The model under review builds one solid part; all positions refer to its coordinate system, in mm. Face numbers are marked on the shaded views. A direction names the side the tool comes from. Give positions to 0.01 mm unless a question says otherwise; leave off trailing zeros. Loops run counter-clockwise (first coordinate to the right, second up) from the corner with the lowest first, then second, coordinate; pieces in that order, holes last. Notation, with made-up numbers: (46.5, 54.25) - (88.5, 54.25) arc R22 cw to (88.5, 60.25) - close; hole circle Ø10 at (-26.5, 71.25). An arc over 180 degrees is marked (long way). Return JSON: item names as keys, results as strings. Group by question number.
from build123d import *

# Parameters (mm, degrees)
SKETCH1_W           = 23
SKETCH1_H           = 12
BOSS_EXTRUDE1_DEPTH = 32
SKETCH2_W           = 4.5
SKETCH2_H           = 2
BOSS_EXTRUDE2_DEPTH = 12
CUT_EXTRUDE1_DEPTH  = 37.912057651
SKETCH4_W           = 23
SKETCH4_H           = 12
SKETCH4_R           = 2.5
CUT_EXTRUDE2_DEPTH  = 3.5
CUT_EXTRUDE3_DEPTH  = 5.5
FILLET1_R           = 1


with BuildPart() as part:
    # Sketch1 → Boss-Extrude1 (new body)
    with BuildSketch(Plane.XY):
        with Locations((11.5, 6)):
            Rectangle(SKETCH1_W, SKETCH1_H)
    extrude(amount=BOSS_EXTRUDE1_DEPTH)

    # Sketch2 → Boss-Extrude2 (add)
    with BuildSketch(Plane.XZ):
        with Locations((-2.25, 20.5)):
            Rectangle(SKETCH2_W, SKETCH2_H)
        with Locations((25.25, 20.5)):
            Rectangle(SKETCH2_W, SKETCH2_H)
    extrude(amount=-BOSS_EXTRUDE2_DEPTH)

    # Sketch3 → Cut-Extrude1 (cut, through all)
    with BuildSketch(Plane.XY.offset(21.5)):
        with BuildLine():
            Line((-3.549038106, 6.75), (-4.5, 6.75))
            Line((-4.5, 6.75), (-4.5, 5.25))
            Line((-4.5, 5.25), (-3.549038106, 5.25))
            ThreePointArc((-3.549038106, 5.25), (-0.75, 6), (-3.549038106, 6.75))
        make_face()
        with BuildLine():
            Line((26.549038106, 6.75), (27.5, 6.75))
            Line((27.5, 6.75), (27.5, 5.25))
            Line((27.5, 5.25), (26.549038106, 5.25))
            ThreePointArc((26.549038106, 5.25), (23.75, 6), (26.549038106, 6.75))
        make_face()
    extrude(amount=-CUT_EXTRUDE1_DEPTH, mode=Mode.SUBTRACT)

    # Sketch4 → Cut-Extrude2 (cut)
    with BuildSketch(Plane.XY.offset(32)):
        with Locations((11.5, 6)):
            Rectangle(SKETCH4_W, SKETCH4_H)
        with Locations((6, 6)):
            Circle(SKETCH4_R, mode=Mode.SUBTRACT)
    extrude(amount=-CUT_EXTRUDE2_DEPTH, mode=Mode.SUBTRACT)

    # Sketch5 → Cut-Extrude3 (cut)
    with BuildSketch(Plane.XY.offset(28.5)):
        with BuildLine():
            ThreePointArc((11.479166667, 3.554855293), (9.2656647, 0.966568361), (6.000000021, 0))
            Line((6.000000021, 0), (23, 0))
            Line((23, 0), (23, 12))
            Line((23, 12), (6.000000023, 12))
            ThreePointArc((6.000000023, 12), (9.265664701, 11.033431639), (11.479166667, 8.445144707))
            ThreePointArc((11.479166667, 8.445144707), (14.5, 6), (11.479166667, 3.554855293))
        make_face()
        with BuildLine():
            Line((0, 12), (0, 6.000000008))
            ThreePointArc((0, 6.000000008), (1.757359324, 10.242640698), (6.000000023, 12))
            Line((6.000000023, 12), (0, 12))
        make_face()
        with BuildLine():
            Line((0, 6.000000008), (0, 0))
            Line((0, 0), (6.000000021, 0))
            ThreePointArc((6.000000021, 0), (1.757359317, 1.757359308), (0, 6.000000008))
        make_face()
    extrude(amount=-CUT_EXTRUDE3_DEPTH, mode=Mode.SUBTRACT)

    # Fillet1
    fillet1_edges = [part.edges().sort_by_distance(p)[0] for p in [
        (23, 6, 0),
        (11.5, 12, 0),
        (0, 6, 0),
        (11.5, 0, 0),
        (27.5, 0, 20.5),
        (27.5, 12, 20.5),
        (-4.5, 12, 20.5),
        (-4.5, 0, 20.5),
        (0, 0, 9.75),
        (23, 0, 9.75),
        (23, 12, 9.75),
        (0, 12, 9.75),
    ]]
    fillet(fillet1_edges, radius=FILLET1_R)


solid = part.part
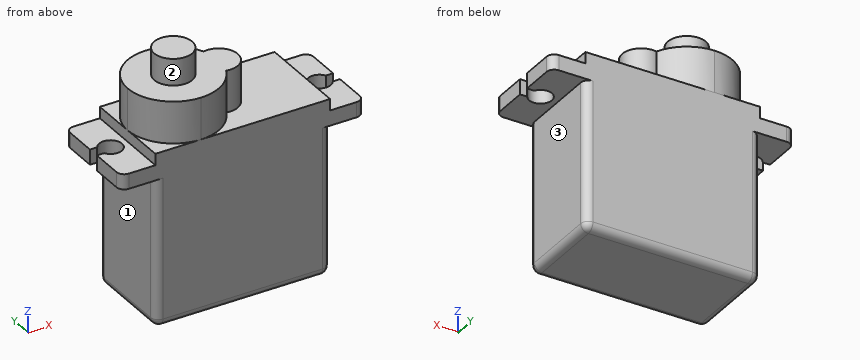
Item 1: Take a section at A-A (x = -2.25). State the section outline as (y, z) points.
Item 2: Tool access review of the marked faces 1, 2 and 3: name each direction out of +Z, -Z, +X, -X, +Y, -Y from which nothing blocks a thin tool from reaching the whole face with its end or side.
Item 3: Take a section at B-B (z = 12.5). State the section outline as (x, y) points, then the cut area to 3 significant figures.
Item 4: Take a section at C-C (x = 12). State the section outline as (y, z) points, then the cut area to 3 significant figures.
Item 5: For L1, parallel to Z at x = 1, y = 10.5; L2, parallel to X at y = 6, z = 20.85, list the stretches that pass through material, from the lowest coordinate up. Write a range as from..to.
Item 6: For P1, Ø6, axis at x = -2, y = 7, coming from the -Z side; P2, Ø5, axis at y = 4.5, z = 8.5, coming from the -X side; P3, Ø1, axis at y = 6, z = 19.5, coming from the +X side; P4, Ø3, axis at x = 1.5, y = 8, coming from the +Z side, all flat-tipped, find the tip position at first contact; note any pin that passes through.
Item 7: Take a section at D-D (y = 2). State the section outline as (x, z) points, then the cut area to 3 significant figures.
Check sheet entries:
{
 "1": {"outline": "(0, 19.5) - (4.5, 19.5) - (4.5, 21.5) - (0, 21.5) - close; (7.5, 19.5) - (12, 19.5) - (12, 21.5) - (7.5, 21.5) - close"},
 "2": {"face 1": "-Z, -X, +Y, -Y", "face 2": "+Z", "face 3": "-Z, +X, +Y, -Y"},
 "3": {"outline": "(0, 1) arc R1 ccw to (1, 0) - (22, 0) arc R1 ccw to (23, 1) - (23, 11) arc R1 ccw to (22, 12) - (1, 12) arc R1 ccw to (0, 11) - close", "area": "275 mm^2"},
 "4": {"outline": "(0, 1) arc R1 ccw to (1, 0) - (11, 0) arc R1 ccw to (12, 1) - (12, 23) - (8.5, 23) - (8.5, 28.5) - (3.5, 28.5) - (3.5, 23) - (0, 23) - close", "area": "303 mm^2"},
 "5": {"L1": "z = 0..23", "L2": "x = -0.75..23.75"},
 "6": {"P1": "stops at z = 0", "P2": "stops at x = 0", "P3": "stops at x = 23.84", "P4": "stops at z = 28.5"},
 "7": {"outline": "(-4.5, 19.5) - (0, 19.5) - (0, 1) arc R1 ccw to (1, 0) - (22, 0) arc R1 ccw to (23, 1) - (23, 19.5) - (27.5, 19.5) - (27.5, 21.5) - (23, 21.5) - (23, 23) - (10.47, 23) - (10.47, 28.5) - (1.53, 28.5) - (1.53, 23) - (0, 23) - (0, 21.5) - (-4.5, 21.5) - close", "area": "596 mm^2"}
}
